For this review, take the finished solid that the model builds, in its own axes (mm). A direction names the side the tool comes from. Give positions to 0.01 mm unless a question says otherwise; leave off trailing zeros. Order: outer loops, then holes, each group sorted by start corner. A loop starts at its lowest first (then second) coordinate and runs counter-clockwise, first axis right, second up. Notation, with made-up numbers: (57, 65) -> (66, 65) arc R17 cw to (66, 72) -> close; hole circle Ø8 at (23.5, -13). An arc over 180 degrees is marked (long way). Return JSON: item names as keys, results as strings. Group by question number.
1) To check wall thickness, follow line 1 along Y through (x, z) = (5.5, 9.5); line 2 along X through (y, z) = (1, 7.25); line 3 along X through (y, z) = (-0.25, 1.75). State the ranges of each line that lie inside material, in increasing order.
2) Insertion check: P1, Ø1.8, axis at x = 0.5, z = 9.5, coming from the +Y side; P2, Ø1, axis at y = 2, z = 14.5, coming from the -X side; P3, Ø1.1, axis at x = 3.5, z = 9, coming from the -Y side. Each pin has a flat end and moves straight along its axis. Give the tip position at first contact, or say it passes through.
3) The part is to be moulded in two halves that separate along X. For faces 6 (the face through (4.54, -0.04, 9.55)), 7 (the face through (0, 2.75, 8.8)), 8 (the face through (-3, 0, 6)), say which applies: released by +X, released by -X, zero draft, split by the parting line, or undercut.
4) Add section C-C (x = -6). Give the boundary of the cut face in (y, z).
5) For faces 1 (the face through (0, -2.75, 8.8)), 2 (the face through (1.3, -1.3, 4)), 3 (the face through (0, 0, 17.093)), 4 (the face through (1.29, -2.024, 10.525)), 5 (the face through (0.01, 2.59, 9)), list the 3-axis set-ups (+Z, -Z, +X, -X, +Y, -Y) from which the entire face can be reached by the end or side of a thin tool; tool diameter is ignored.
6) Add section A-A (z = 9.25). Give the boundary of the cut face in (x, y).
7) Add section B-B (z = 3). Give the boundary of the cut face in (x, y).
8) Add section D-D (z = 14). Give the boundary of the cut face in (x, y), then the cut area to 3 significant figures.
Autodesk Inventor part; units mm, degrees
ref_plane "YZ Plane" through (0, 0, 0) normal (1, 0, 0) x (0, 1, 0)
ref_plane "XZ Plane" through (0, 0, 0) normal (0, 1, 0) x (-1, 0, 0)
ref_plane "XY Plane" through (0, 0, 0) normal (0, 0, 1) x (1, 0, 0)
sketch "Sketch1" plane through (0, 0, 0) normal (0, 1, 0) x (-1, 0, 0)
  line L0 (0, 0) -> (0, 17.0928)
  line L1 (0, 17.0928) -> (-0.9185, 17.0928)
  line L2 (-0.9185, 17.0928) -> (-3.25, 12.0928)
  line L3 (-3.25, 12.0928) -> (-2.4, 12.0928)
  line L4 (-2.4, 12.0928) -> (-2.4, 8.2928)
  line L5 (-2.4, 8.2928) -> (-3, 8.2928)
  line L6 (-3, 8.2928) -> (-3, 4)
  line L7 (-3, 4) -> (-1.5, 4)
  line L8 (-1.5, 4) -> (-1.5, 0)
  line L9 (-1.5, 0) -> (0, 0)
  arc A0 (-6.8684, 10.0226) -> (0, 8.2928) centre (0, 22.7935) ccw
  arc A1 (-6.6316, 10.4629) -> (-2.4, 9) centre (0, 22.7935) ccw
  arc A2 (-6.6316, 10.4629) -> (-6.8684, 10.0226) centre (-6.75, 10.2428) ccw
  line L10 (-2.4, 9) -> (0, 9)
  point P0 (0, 10)
  dimension "d0" = 3
  dimension "d1" = 4
  dimension "d3" = 6
  dimension "d4" = 5
  dimension "d5" = 6.5
  dimension "d9" = 8.8
  dimension "d10" = 25
  dimension "d11" = 4.8
  dimension "d15" = 5
  dimension "d17" = 14
  dimension "d18" = 0.5
  dimension "d19" = 1.6
revolve "Revolution1" add sketch "Sketch1" angle 360 about axis through (0, 0, 0) along (0, 0, 1) contours L9 L8 L7 L6 L5 L4 A0 L0 | A0 L4 L10 L0 | L10 L4 L3 L2 L1 L0
extrude "Extrusion1" add sketch "Sketch1" along normal mid plane 5.5 contours A0 L4 L10 L0 | A0 A2 A1 L4
mirror "Mirror1" about plane through (0, 0, 8.2928) normal (-1, 0, 0) of "Extrusion1"
properties part number "WBN-305" material "Acetal Resin, White"
Evaluation:
{
 "1": {"line 1": "-2.75 to 2.75", "line 2": "-2.83 to 2.83", "line 3": "-1.48 to 1.48"},
 "2": {"P1": "y = 2.75", "P2": "x = -1.61", "P3": "y = -2.75"},
 "3": {"face 6": "undercut", "face 7": "zero draft", "face 8": "split by the parting line"},
 "4": {"outline": "(-2.75, 9.59) -> (2.75, 9.59) -> (2.75, 10.14) -> (-2.75, 10.14) -> close"},
 "5": {"face 1": "+X, -X, -Y", "face 2": "-Z", "face 3": "+Z, +X, -X, +Y, -Y", "face 4": "none", "face 5": "+Y"},
 "6": {"outline": "(-5.18, -2.75) -> (-3.55, -2.75) -> (-3.55, 2.75) -> (-5.18, 2.75) -> close; circle Ø4.8 at (0, 0); (3.55, -2.75) -> (5.18, -2.75) -> (5.18, 2.75) -> (3.55, 2.75) -> close"},
 "7": {"outline": "circle Ø3 at (0, 0)"},
 "8": {"outline": "circle Ø4.72 at (0, 0)", "area": "17.5 mm^2"}
}
